The listing builds one solid part. Answer for the finished solid, in the listing's coordinates (mm). A direction names the side the tool comes from. Round coordinates to 2 decimals unless told otherwise and drop trailing zeros. Order: outer loops, then holes, each group sorted by start corner. A loop starts at its lowest first (then second) coordinate and runs counter-clockwise, first axis right, second up. Notation, with made-up numbers: (0.25, -37) -> (55.25, -37) arc R27 cw to (55.25, -21) -> close; hole circle Ø9 at (66, 37). An arc over 180 degrees is marked (long way). Return JSON: item names as keys, results as strings. Group by question number.
(1) The part is cut by section D-D (z = 55). Determine the outline of the cut face in (x, y) (3 decimals), plus the area to 3 significant figures.
(2) Each of these flat-tipped pins is pushed along its axis until it touches: pin 1 (1 mm diameter, centred on x = -34, y = 3.5, fed in from -Z); pin 2 (3.5 mm diameter, centred on x = -23.5, z = 31, fed in from +Y); pin 3 (6.5 mm diameter, centred on y = -14.5, z = 250.5, fed in from -X); pin 4 (10 mm diameter, centred on x = 4.5, y = -7, fed in from +Z). Where does it stop, or does it pass through?
(3) The part is cut by section B-B (y = -13.5). Determine the outline of the cut face in (x, z) (3 decimals), plus the area to 3 significant figures.
(4) The part is cut by section A-A (z = 101.7). Determine the outline of the cut face in (x, y) (3 decimals).
(5) Determine the mould class of faces 6 (the face through (-27, -22.25, 250)), 7 (the face through (0, 24, 27.45)), 8 (the face through (21.73, 19.474, 45.143)), 9 (the face through (-35, 11, 84)) for opening direction X: +X half, -X half, draft (parallel to the pull), parting line (faces both ways), or undercut.
(6) Which of the six approach directions +Z, -Z, +X, -X, +Y, -Y give full straight-line access (tool end or side, diameter ignored) to faces 1 (the face through (0, 24, 31.95)), 2 (the face through (-22.11, 19.474, 132.803)), 3 (the face through (29, 22.25, 199)), 4 (the face through (0, 23.7, 141)), 5 (the face through (0, 10, 24.7))?
(7) The part is cut by section C-C (x = 0). Count the separate pieces of the cut face and the enclosed holes in it, plus the area to 3 significant figures.
(8) Consider line 1 (Z direction, x = -29, y = 2.5); line 2 (Z direction, x = -32.4, y = 9.7); line 3 (Z direction, x = 0, y = 23). Determine where each line is inside the solid, lowest interval first. Write a range as [from, to].
from build123d import *

# Parameters (mm, degrees)
PAD017_DEPTH    = 4.5
SKETCH028_W     = 50.8
SKETCH028_H     = 15
PAD024_DEPTH    = 10
PAD021_DEPTH    = 100.98
SKETCH025_R     = 3.8
PAD022_DEPTH    = 3.5
SKETCH026_R     = 1.8
PAD023_DEPTH    = 1.5
SKETCH042_R     = 8
POCKET002_DEPTH = 5
PAD031_DEPTH    = 4.5
SKETCH034_W     = 70
SKETCH034_H     = 24.7
PAD030_DEPTH    = 10
SKETCH037_W     = 10
SKETCH037_H     = 10
PAD033_DEPTH    = 110.5
SKETCH038_W     = 10
SKETCH038_H     = 10
PAD034_DEPTH    = 34.5
SKETCH039_W     = 10
SKETCH039_H     = 10
PAD035_DEPTH    = 34.5
SKETCH040_W     = 22.25
SKETCH040_H     = 110.5
PAD036_DEPTH    = 3.5
PAD016_DEPTH    = 70
CHAMFER010_SIZE = 2.125
CHAMFER012_SIZE = 2.125
SKETCH044_R     = 5.5
SKETCH044_W     = 7
SKETCH044_H     = 12
POCKET004_DEPTH = 5


with BuildPart() as band2:
    # Sketch020 → Pad017 (new body)
    with BuildSketch(Plane.XY.offset(27.45)):
        Polygon((-35, 24.7), (-35, 0), (-34, 0), (-34, 23.7), (-20, 23.7), (-20, 22.7), (20, 22.7), (20, 23.7), (34, 23.7), (34, 0), (35, 0), (35, 24.7), align=None)
    extrude(amount=PAD017_DEPTH)


with BuildPart() as body012:
    # Sketch028 → Pad024 (new body)
    with BuildSketch(Plane.XZ.offset(-24.7)):
        with Locations((0, 119.38)):
            Rectangle(SKETCH028_W, SKETCH028_H)
    extrude(amount=PAD024_DEPTH)


with BuildPart() as boardbacking:
    # Sketch024 → Pad021 (new body)
    with BuildSketch(Plane.XY.offset(34.7)):
        Polygon((-35, 0), (-35, 24.7), (35, 24.7), (35, 0), (31.5, 0), (31.5, 21.2), (-31.5, 21.2), (-31.5, 0), align=None)
    extrude(amount=PAD021_DEPTH)

    # Sketch025 (on Face6 of Pad021) → Pad022 (join)
    with BuildSketch(Plane.XZ.offset(-21.2)):
        with Locations((-22.225, 129.005)):
            Circle(SKETCH025_R)
        with Locations((22.225, 129.005)):
            Circle(SKETCH025_R)
        with Locations((-22.225, 41.375)):
            Circle(SKETCH025_R)
        with Locations((22.225, 41.375)):
            Circle(SKETCH025_R)
    extrude(amount=PAD022_DEPTH)

    # Sketch026 → Pad023 (join)
    with BuildSketch(Plane.XZ.offset(-17.7)):
        with Locations((-22.225, 129.005)):
            Circle(SKETCH026_R)
        with Locations((22.225, 129.005)):
            Circle(SKETCH026_R)
        with Locations((-22.225, 41.375)):
            Circle(SKETCH026_R)
        with Locations((22.225, 41.375)):
            Circle(SKETCH026_R)
    extrude(amount=PAD023_DEPTH)

    # Boolean005: cut Body012
    add(body012.part, mode=Mode.SUBTRACT)

    # Sketch042 (on Face3 of Boolean005) → Pocket002 (cut)
    with BuildSketch(Plane(origin=(0, 24.7, 0), x_dir=(-1, 0, 0), z_dir=(0, 1, 0))):
        with Locations((0, 55)):
            Circle(SKETCH042_R)
        with BuildLine():
            Line((3.641143, 64.313543), (18.302914, 86.985827))
            Line((18.302914, 86.985827), (21.661771, 84.813713))
            Line((21.661771, 84.813713), (7, 62.141428))
            ThreePointArc((7, 62.141428), (5.430286, 63.397142), (3.641143, 64.313543))
        make_face()
        with BuildLine():
            ThreePointArc((15.712042, 88.498235), (3.658274, 91.818705), (-8.813211, 90.935043))
            Line((-9.765986, 94.819914), (-8.813211, 90.935043))
            Line((-21.351919, 86.31544), (-9.765986, 94.819914))
            Line((-7.145856, 84.136519), (-21.351919, 86.31544))
            Line((-8.098631, 88.02139), (-7.145856, 84.136519))
            ThreePointArc((14.438081, 85.782167), (3.361649, 88.833405), (-8.098631, 88.02139))
            Line((15.712042, 88.498235), (14.438081, 85.782167))
        make_face()
    extrude(amount=-POCKET002_DEPTH, mode=Mode.SUBTRACT)


with BuildPart() as body017:
    # Sketch035 → Pad031 (new body)
    with BuildSketch(Plane.XY.offset(138.43)):
        Polygon((-35, 0), (-35, 24.7), (35, 24.7), (35, 0), (34, 0), (34, 23.7), (-34, 23.7), (-34, 0), align=None)
    extrude(amount=PAD031_DEPTH)


with BuildPart() as zip003:
    # Sketch034 → Pad030 (new body)
    with BuildSketch(Plane.XY.offset(135.68)):
        with Locations((0, 12.35)):
            Rectangle(SKETCH034_W, SKETCH034_H)
    extrude(amount=PAD030_DEPTH)

    # Boolean007: cut Body017
    add(body017.part, mode=Mode.SUBTRACT)

    # Sketch037 (on Face12 of Boolean007) → Pad033 (join)
    with BuildSketch(Plane.XY.offset(145.68)):
        with Locations((-26.5, 17.25)):
            Rectangle(SKETCH037_W, SKETCH037_H)
        with Locations((26.5, 17.25)):
            Rectangle(SKETCH037_W, SKETCH037_H)
    extrude(amount=PAD033_DEPTH)

    # Sketch038 (on Face21 of Pad033) → Pad034 (join)
    with BuildSketch(Plane.XZ.offset(-12.25)):
        with Locations((-26.5, 251.18)):
            Rectangle(SKETCH038_W, SKETCH038_H)
    extrude(amount=PAD034_DEPTH)

    # Sketch039 (on Face17 of Pad034) → Pad035 (join)
    with BuildSketch(Plane.XZ.offset(-12.25)):
        with Locations((26.5, 251.18)):
            Rectangle(SKETCH039_W, SKETCH039_H)
    extrude(amount=PAD035_DEPTH)

    # Sketch040 (on Face22 of Pad035) → Pad036 (join)
    with BuildSketch(Plane(origin=(-31.5, 0, 0), x_dir=(0, -1, 0), z_dir=(-1, 0, 0))):
        with Locations((-11.125, 200.93)):
            Rectangle(SKETCH040_W, SKETCH040_H)
    pad036 = extrude(amount=PAD036_DEPTH)

    # Mirrored: Pad036 across YZ
    add(pad036.mirror(Plane.YZ))


with BuildPart() as frame:
    # Sketch019 → Pad016 (new body)
    with BuildSketch(Plane.YZ.offset(-35)):
        Polygon((0, 34.7), (0, 24.7), (20.45, 24.7), (24.7, 20.45), (24.7, 34.7), align=None)
    extrude(amount=PAD016_DEPTH)

    # Boolean004: cut Band2
    add(band2.part, mode=Mode.SUBTRACT)

    # Boolean008: union BoardBacking, Zip003
    add(boardbacking.part)
    add(zip003.part)

    # Chamfer010
    chamfer010_edges = [frame.edges().sort_by_distance(p)[0] for p in [
        (35, 24.7, 23.95),
        (34, 23.7, 29.7),
        (35, 24.7, 33.325),
        (35, 24.7, 85.19),
        (35, 24.7, 137.055),
        (34, 23.7, 140.68),
        (35, 24.7, 144.305),
        (-35, 24.7, 144.305),
        (-34, 23.7, 140.68),
        (-35, 24.7, 137.055),
        (-35, 24.7, 85.19),
        (-35, 24.7, 33.325),
        (-34, 23.7, 29.7),
        (-35, 24.7, 23.95),
    ]]
    chamfer(chamfer010_edges, length=CHAMFER010_SIZE)

    # Chamfer012
    chamfer012_edges = [frame.edges().sort_by_distance(p)[0] for p in [
        (31.5, -22.25, 251.18),
        (31.5, -11.125, 256.18),
        (26.5, -22.25, 256.18),
        (21.5, -22.25, 251.18),
        (21.5, -5, 256.18),
        (21.5, 17.25, 256.18),
        (26.5, 22.25, 256.18),
        (33.25, 22.25, 256.18),
        (21.5, 22.25, 200.93),
        (-21.5, 22.25, 200.93),
        (-26.5, 22.25, 256.18),
        (-33.25, 22.25, 256.18),
        (-21.5, 17.25, 256.18),
        (-21.5, -5, 256.18),
        (-21.5, -22.25, 251.18),
        (-31.5, -22.25, 251.18),
        (-26.5, -22.25, 256.18),
        (-31.5, -11.125, 256.18),
    ]]
    chamfer(chamfer012_edges, length=CHAMFER012_SIZE)

    # Sketch044 (on Face54 of Chamfer012) → Pocket004 (cut)
    with BuildSketch(Plane(origin=(-35, 0, 0), x_dir=(0, -1, 0), z_dir=(-1, 0, 0))):
        with Locations((-9.7, 101.7)):
            Circle(SKETCH044_R)
        with Locations((-2.34, 81.38)):
            Rectangle(SKETCH044_W, SKETCH044_H)
    extrude(amount=-POCKET004_DEPTH, mode=Mode.SUBTRACT)


solid = frame.part
Answer below:
{
 "1": {"outline": "(-35, 0) -> (-31.5, 0) -> (-31.5, 21.2) -> (-8, 21.2) -> (-8, 24.7) -> (-32.875, 24.7) -> (-35, 22.575) -> close; (8, 21.2) -> (31.5, 21.2) -> (31.5, 0) -> (35, 0) -> (35, 22.575) -> (32.875, 24.7) -> (8, 24.7) -> close", "area": "333 mm²"},
 "2": {"pin 1": "stops at z = 24.7", "pin 2": "stops at y = 24.7", "pin 3": "stops at x = -31.5", "pin 4": "passes through"},
 "3": {"outline": "(-31.5, 246.18) -> (-21.5, 246.18) -> (-21.5, 254.055) -> (-23.625, 256.18) -> (-29.375, 256.18) -> (-31.5, 254.055) -> close; (21.5, 246.18) -> (31.5, 246.18) -> (31.5, 254.055) -> (29.375, 256.18) -> (23.625, 256.18) -> (21.5, 254.055) -> close", "area": "191 mm²"},
 "4": {"outline": "(-35, 0) -> (-31.5, 0) -> (-31.5, 4.2) -> (-35, 4.2) -> close; (-35, 15.2) -> (-31.5, 15.2) -> (-31.5, 21.2) -> (31.5, 21.2) -> (31.5, 0) -> (35, 0) -> (35, 22.575) -> (32.875, 24.7) -> (-32.875, 24.7) -> (-35, 22.575) -> close"},
 "5": {"face 6": "draft", "face 7": "undercut", "face 8": "undercut", "face 9": "-X half"},
 "6": {"face 1": "+Y", "face 2": "-Y", "face 3": "+Z, +X, -X, +Y", "face 4": "+X, -X, +Y", "face 5": "-Z, +X, -X, -Y"},
 "7": {"separate pieces": "4", "enclosed holes": "0", "area": "724 mm²"},
 "8": {"line 1": "z = [24.7, 34.7], [135.68, 145.68], [246.18, 256.18]", "line 2": "z = [24.7, 96.2], [107.2, 256.18]", "line 3": "z = [22.15, 27.45], [31.95, 47], [63, 89], [92, 111.88], [126.88, 145.68]"}
}
